Can you work these out from the drawing? Everything is in mm from the part's minimum corner. Give positions to 0.01 mm unless a question says otherwise; leave off trailing zeros. Order: outer loops, then holes, each group sorted by start corner. A loop starts at its lowest first (then second) coordinate and runs counter-clockwise, first axis right, second up. Notation, with made-up numbers: (78.25, 54) - (114.25, 54) arc R15 cw to (114.25, 81) - close; hole circle Ø11 at (55, -39). An arc over 180 degrees is marked (long way). One line per question, with ' | ' between items.
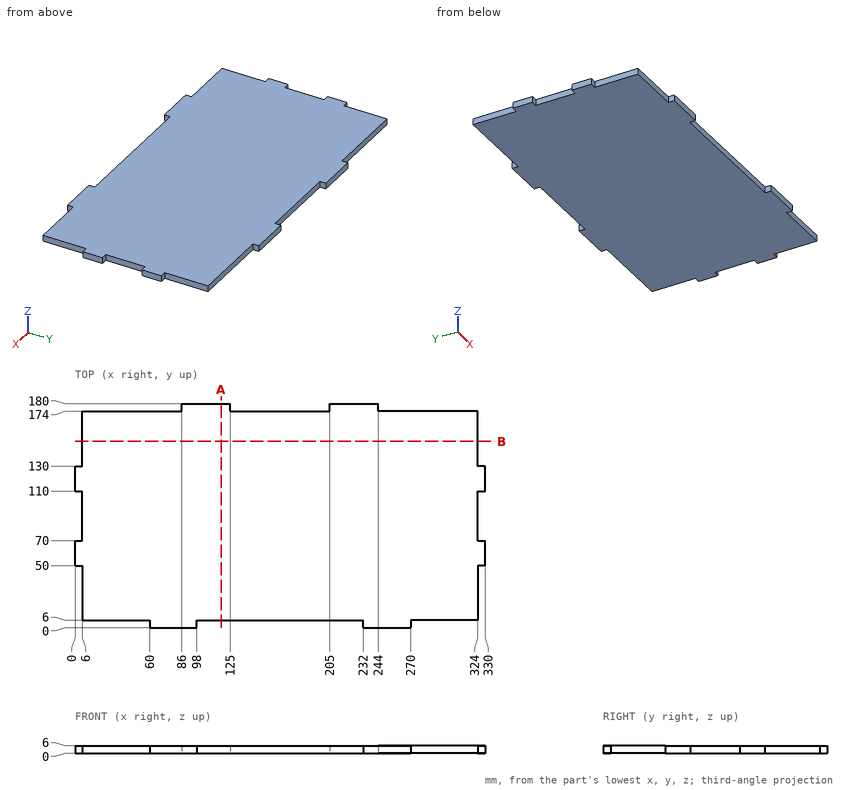
(1) Will these pins go through, and if not, where does the flat tip stop? pin 1 (1.8 mm diameter, centred on y = 4, z = 3.5, fed in from -X); pin 2 (1.8 mm diameter, centred on y = 176, z = 4, fed in from +X); pin 3 (3 mm diameter, centred on y = 96.5, z = 3, fed in from -X).
Answer below:
pin 1: x = 60 | pin 2: x = 244 | pin 3: x = 6
(2) Imagine slicing it at B-B (y = 150). List the corners of the cut face in (x, z) for me, and give its area (3 significant figures).
Answer below:
outline: (6, 0) - (324, 0) - (324, 6) - (6, 6) - close | area: 1,910 mm^2
(3) If I drill on line 1 (X direction, y = 74, z = 2.3); line 2 (Y direction, x = 198.5, z = 4); line 3 (Y direction, x = 206, z = 2.05), over which ranges is the centre line in solid material (lowest first)?
Answer below:
line 1: 6 to 324 | line 2: 6 to 174 | line 3: 6 to 180
(4) Imagine slicing it at A-A (x = 117.5). List the corners of the cut face in (y, z) for me.
Answer below:
outline: (6, 0) - (180, 0) - (180, 6) - (6, 6) - close
